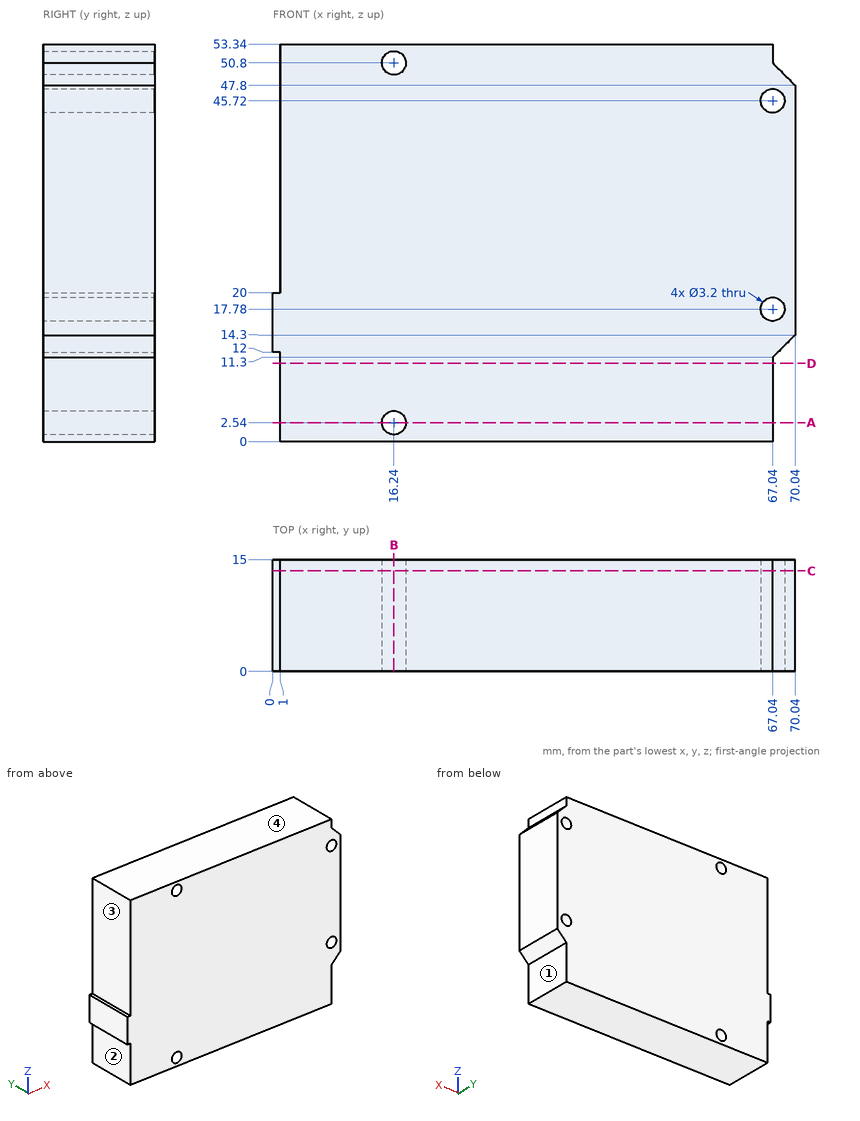
Design review of the part shown in the three views and the two pictorial views. Dimensions are in mm from the part's minimum x, y and z. A direction names the side the tool comes from. Give positions to 0.01 mm unless a question says otherwise; leave off trailing zeros. Order: outer loops, then holes, each group sorted by start corner. A loop starts at its lowest first (then second) coordinate and runs counter-clockwise, first axis right, second up. Notation, with made-up numbers: M -6.75,74 L 41.25,74 A7 cw 41.25,84 Z; hole C -7,-12 d3. An arc over 180 degrees is marked long. Answer in a Markdown table with one row per item. Add a question column.
(1) Consider section B-B on x = 16.24. State the section outline as (y, z) points.
(2) Wall thickness on probe 1 along X at (y, z) = (8.75, 2.54); probe 2 along X at (y, z) = (11.75, 18); probe 3 along X at (y, z) = (12.5, 42): over which ranges is each line inside the solid? List them lowest first. Write a range as [from, to].
(3) Consider section A-A on z = 2.54. State the section outline as (x, y) points.
(4) For pin 1 (1.5 mm diameter, centred on x = 12.5, z = 7.5, fed in from -Y); pin 2 (3 mm diameter, centred on y = 8, z = 51.5, fed in from +X); pin 3 (9 mm diameter, centred on y = 5.5, z = 6, fed in from +X), all flat-tipped, find the tip position at first contact; note any pin that passes through.
(5) Consider section D-D on z = 10.5. State the section outline as (x, y) points, and give its area (3 significant figures).
(6) Consider section C-C on y = 13.5. State the section outline as (x, z) points.
(7) For the marked faces 1, 2, 3 and 4, list the 3-axis set-ups (+Z, -Z, +X, -X, +Y, -Y) from which the entire face can be reached by the end or side of a thin tool; tool diameter is ignored.
Evaluation:
| question | item | result |
|---|---|---|
| 1 | outline | M 0,0 L 15,0 L 15,0.94 L 0,0.94 Z; M 0,4.14 L 15,4.14 L 15,49.2 L 0,49.2 Z; M 0,52.4 L 15,52.4 L 15,53.34 L 0,53.34 Z |
| 2 | probe 1 | x = [1, 14.64], [17.84, 67.04] |
| 2 | probe 2 | x = [0, 65.46], [68.62, 70.04] |
| 2 | probe 3 | x = [1, 70.04] |
| 3 | outline | M 1,0 L 14.64,0 L 14.64,15 L 1,15 Z; M 17.84,0 L 67.04,0 L 67.04,15 L 17.84,15 Z |
| 4 | pin 1 | stops at y = 0 |
| 4 | pin 2 | stops at x = 67.84 |
| 4 | pin 3 | stops at x = 67.04 |
| 5 | outline | M 1,0 L 67.04,0 L 67.04,15 L 1,15 Z |
| 5 | area | 991 mm^2 |
| 6 | outline | M 0,12 L 1,12 L 1,0 L 67.04,0 L 67.04,11.3 L 70.04,14.3 L 70.04,47.8 L 67.04,50.8 L 67.04,53.34 L 1,53.34 L 1,20 L 0,20 Z; hole C 16.24,2.54 d3.2; hole C 16.24,50.8 d3.2; hole C 67.04,17.78 d3.2; hole C 67.04,45.72 d3.2 |
| 7 | face 1 | -Z, +X, +Y, -Y |
| 7 | face 2 | -Z, -X, +Y, -Y |
| 7 | face 3 | +Z, -X, +Y, -Y |
| 7 | face 4 | +Z, +X, -X, +Y, -Y |
